from build123d import *

# Parameters (mm, degrees)
F0_W     = 127
F0_H     = 127
F1_DEPTH = 152.4
F3_DEPTH = 101.6
F4_R     = 7.6138039838
F4_R_2   = 7.6607113174
F5_DEPTH = 203.2
F6_T     = -2.54


with BuildPart() as f1:
    # F0 (on Top) → F1 (new body)
    with BuildSketch(Plane.XY):
        with Locations((4.3386593461, -2.4487966104)):
            Rectangle(F0_W, F0_H)
    extrude(amount=F1_DEPTH)

    # F2 (on face) → F3 (cut)
    with BuildSketch(Plane.XY.offset(152.4)):
        Polygon((-8.3613406539, 61.0512033896), (-59.1613406539, 61.0512033896), (-59.1613406539, 10.2512033896), align=None)
        Polygon((67.8386593461, -15.1487966104), (17.0386593461, -65.9487966104), (67.8386593461, -65.9487966104), align=None)
    extrude(amount=-F3_DEPTH, mode=Mode.SUBTRACT)

    # F4 (on face) → F5 (cut)
    with BuildSketch(Plane.XY.offset(50.8)):
        with Locations((-45.811150223, 46.3215783238)):
            Circle(F4_R)
        with Locations((50.4050254822, -53.2123930752)):
            Circle(F4_R_2)
    extrude(amount=-F5_DEPTH, mode=Mode.SUBTRACT)

    # F6
    f6_openings = [f1.faces().sort_by_distance(p)[0] for p in [
        (4.379261, -2.418518, 0),
    ]]
    offset(amount=F6_T, openings=f6_openings, kind=Kind.INTERSECTION)


solid = f1.part
Design review of the part built by this model. Coordinates are the model's own, in mm. A direction names the side the tool comes from. Coordinates: 2 decimals unless noted, no trailing zeros. Loops run counter-clockwise (first coordinate to the right, second up) from the corner with the lowest first, then second, coordinate; pieces in that order, holes last. Notation, with made-up numbers: M 45.25,62.5 L 64.25,62.5 A29 ccw 64.25,86.5 Z; hole C 10,61.5 d10. An arc over 180 degrees is marked long. Use one line per item in the form item = value.
(1) Consider section D-D (z = 36.5). Write out the cut boundary in (x, y), and give its area (3 significant figures).
Return value:
outline = M -59.16,-65.95 L 67.84,-65.95 L 67.84,61.05 L -59.16,61.05 Z; C -45.81,46.32 d20.31; hole M -56.62,-63.41 L 50.11,-63.41 A10.2 cw long 50.7,-63.41 L 65.3,-63.41 L 65.3,58.51 L -56.62,58.51 Z; hole C -45.81,46.32 d15.23; hole C 50.41,-53.21 d15.32
area = 1,550 mm2
(2) Consider section C-C (y = 49). Write out the cut boundary in (x, z).
Return value:
outline = M -59.16,0 L -56.62,0 L -56.62,48.26 L -55.61,48.26 L -55.61,0 L -52.94,0 L -52.94,50.8 L -59.16,50.8 Z; M -38.68,0 L -36.02,0 L -36.02,48.26 L -16.82,48.26 L -16.82,149.86 L 65.3,149.86 L 65.3,0 L 67.84,0 L 67.84,152.4 L -20.41,152.4 L -20.41,50.8 L -38.68,50.8 Z
(3) Consider section B-B (z = 137). Write out the cut boundary in (x, y), and give its area (3 significant figures).
Return value:
outline = M -59.16,-65.95 L 17.04,-65.95 L 67.84,-15.15 L 67.84,61.05 L -8.36,61.05 L -59.16,10.25 Z; hole M -56.62,-63.41 L 15.99,-63.41 L 65.3,-14.1 L 65.3,58.51 L -7.31,58.51 L -56.62,9.2 Z
area = 1,120 mm2
(4) For line 1 along X through (y, z) = (15.5, 40.5); line 2 along Y through (x, z) = (-19, 27); line 3 along Z through (x, y) = (8, 38.5), list the stretches that pass through material, from the lowest coordinate up. Write a range as from..to.
Return value:
line_1 = -59.16..-56.62, 65.3..67.84
line_2 = -65.95..-63.41, 58.51..61.05
line_3 = 149.86..152.4
(5) Consider section A-A (x = 54). Write out the cut boundary in (y, z), and give its area (3 significant figures).
Return value:
outline = M -65.95,0 L -63.41,0 L -63.41,48.26 L -62.76,48.26 L -62.76,0 L -59.98,0 L -59.98,50.8 L -65.95,50.8 Z; M -46.45,0 L -43.67,0 L -43.67,48.26 L -25.4,48.26 L -25.4,149.86 L 58.51,149.86 L 58.51,0 L 61.05,0 L 61.05,152.4 L -28.99,152.4 L -28.99,50.8 L -46.45,50.8 Z
area = 1,420 mm2
(6) For faces 1 (the face through (44.326, -57.874, 25.756)), 2 (the face through (-55.955, 46.768, 24.468)), 3 (the face through (-34, 42, 50.8)), list the 3-axis set-ups (+Z, -Z, +X, -X, +Y, -Y) from which the entire face can be reached by the end or side of a thin tool; tool diameter is ignored.
Return value:
face_1 = +Z, -Z
face_2 = -Z
face_3 = +Z, -X, +Y
(7) Draft analysis for pull direction Y (two halves, no side actions). For faces 4 (the face through (-57, 21, 0)), 5 (the face through (-56.621, -17, 57)), 6 (the face through (42.794, -40.193, 102.311)), 7 (the face through (-46.8, 53.87, 25.76)), state which applies: pulls with the +Y half, pulls with the -Y half, needs draft (parallel to the pull), parting line crosses it, or undercut.
Return value:
face_4 = needs draft
face_5 = undercut
face_6 = pulls with the -Y half
face_7 = undercut
(8) Clearance check with flat-ended pins moving along their axes: P1, Ø5, axis at y = 30.5, z = 77, coming from the -X side; P2, Ø2, axis at x = 42.5, y = 43, coming from the -Z side; P3, Ø4, axis at y = 38, z = 58, coming from the -X side. State where each tip first meets the part, or that it passes through.
Return value:
P1 = -41.41
P2 = 149.86
P3 = -33.41
